from build123d import *

# Parameters (mm, degrees)
F1_DEPTH = 6
F2_R     = 6
F3_DEPTH = 5.5
F4_R     = 4
F5_DEPTH = 11.501
F6_R     = 1


with BuildPart() as f1:
    # F0 (on Top) → F1 (new body)
    with BuildSketch(Plane.XY):
        Polygon((6.85, -3.954849), (6.85, 3.954849), (0, 7.909699), (-6.85, 3.954849), (-6.85, -3.954849), (0, -7.909699), align=None)
    extrude(amount=F1_DEPTH)

    # F2 (on face) → F3 (join)
    with BuildSketch(Plane.XY.offset(6)):
        Circle(F2_R)
    extrude(amount=F3_DEPTH)

    # F4 (on face) → F5 (cut, through all)
    with BuildSketch(Plane.XY.offset(11.5)):
        with Locations((1.8, 0)):
            Circle(F4_R)
    extrude(amount=-F5_DEPTH, mode=Mode.SUBTRACT)

    # F6
    f6_edges = [f1.edges().sort_by_distance(p)[0] for p in [
        (6.85, -3.954849, 3),
        (0, -7.909699, 3),
        (6.85, 3.954849, 3),
        (-6.85, -3.954849, 3),
        (-6.85, 3.954849, 3),
        (0, 7.909699, 3),
    ]]
    fillet(f6_edges, radius=F6_R)


solid = f1.part
Geometry: final body of the model. Coordinates: model frame, mm. A direction names the side the tool comes from. Round coordinates to 2 decimals unless told otherwise and drop trailing zeros. Loops run counter-clockwise (first coordinate to the right, second up) from the corner with the lowest first, then second, coordinate; pieces in that order, holes last. Notation, with made-up numbers: M 84,67 L 134,67 A26 cw 134,105 Z; hole C 72.5,-17.5 d3. An arc over 180 degrees is marked long. Put each result on its own line as item: value. Start each with the question number.
(1) Draft query along Y for faces 1 (the face through (6.85, 0, 3)), 2 (the face through (3.646, -3.549, 5.83)), 3 (the face through (6.72, -3.87, 3.04)). Return one class per face: +Y half, -Y half, draft (parallel to the pull), parting line (faces both ways), or undercut.
(2) Section query B-B (x = -1.75). Return loops of the section in (y, z).
(3) Material intervals for line 1 along Z through (x, y) = (0, -6.75); line 2 along Y through (x, z) = (1.8, 4.5); line 3 along X through (y, z) = (3.25, 9), sorted ascending. Write a range as [from, to].
(4) Section query C-C (y = 0). Return loops of the section in (x, z).
(5) Contact query for flat-ended pins moving along their axis: pin 1 Ø2 at (y, z) = (0.5, 9) entering from +X; pin 2 Ø1 at (y, z) = (5.5, 2.5) entering from +X; pin 3 Ø8 at (x, y) = (4.5, 1.5) entering from +Z; pin 4 Ø6 at (y, z) = (-0.5, 9.5) entering from -X. Output: stop coordinate, or through.
(6) Section query D-D (z = 11.25). Return loops of the section in (x, y).
(7) Set-up query: faces 4 (the face through (3.38, -5.96, 2.96)), 5 (the face through (-2, 6, 6)). Return all of +Z, -Z, +X, -X, +Y, -Y with unobstructed straight access to the full face (end or side cutting, diameter ignored); none if empty.
Findings below:
1. face 1: draft
1. face 2: undercut
1. face 3: -Y half
2. outline: M -6.9,0 L -1.84,0 L -1.84,11.5 L -5.74,11.5 L -5.74,6 L -6.9,6 Z; M 1.84,0 L 6.9,0 L 6.9,6 L 5.74,6 L 5.74,11.5 L 1.84,11.5 Z
3. line 1: z = [0, 6]
3. line 2: y = [-6.87, -4], [4, 6.87]
3. line 3: x = [-5.04, -0.53], [4.13, 5.04]
4. outline: M -6.85,0 L -2.2,0 L -2.2,11.5 L -6,11.5 L -6,6 L -6.85,6 Z; M 5.8,0 L 6.85,0 L 6.85,6 L 6,6 L 6,11.5 L 5.8,11.5 Z
5. pin 1: stops at x = 6
5. pin 2: stops at x = 5.04
5. pin 3: stops at z = 11.5
5. pin 4: stops at x = -6
6. outline: C 0,0 d12; hole C 1.8,0 d8
7. face 4: +Z, -Z, +X, -Y
7. face 5: +Z
